Geometry: final body of the model. Coordinates: model frame, mm. A direction names the side the tool comes from. Give positions to 0.01 mm unless a question says otherwise; leave off trailing zeros. Write each loop counter-clockwise with the first axis right and the second up, starting at its lowest first coordinate (ties: lowest second). Pieces come first, ordered by that corner, then holes. Notation, with made-up numbers: M -38,11.25 L 13,11.25 A14 ccw 13,21.25 Z; hole C -8.75,55 d8. An arc over 180 degrees is marked long. Use a Markdown table: item, result. Add a question column.
1) Pin query (flat end, axial travel): pin 1 (1 mm diameter, centred on x = -36.5, z = 18.5, fed in from +Y); pin 2 (1.8 mm diameter, centred on x = 0.5, y = 0.5, fed in from +Z); pin 3 (1.6 mm diameter, centred on x = -37, y = -2, fed in from +Z). Return the tip coordinate at first contact, or that it passes through.
2) Section D-D on y = -12.5. Return the cut outline in (x, z), then the cut area to 3 significant figures.
3) Line query: line 1 (Y direction, x = -20, z = 24); line 2 (X direction, y = -23, z = 6); line 3 (Z direction, x = -0.5, y = 7). Output: solid intervals per line, ascending.
4) Set-up query: faces 1 (the flat face through (-1, 1, 0)), 2 (the flat face through (37.5, 1, 15)), 3 (the flat face through (-37, -20.029, 15)), 4 (the flat face through (0, 1, 2)), 5 (the flat face through (0, 0, 37)). Return all of +Z, -Z, +X, -X, +Y, -Y with unobstructed straight access to the full face (end or side cutting, diameter ignored); none if empty.
5) Draft query along X for faces 6 (the flat face through (-37.5, -0.6, 4.8)), 7 (the flat face through (-37, 12.126, 15)), 8 (the flat face through (35.5, 1, 15)). Return one class per face: +X half, -X half, draft (parallel to the pull), parting line (faces both ways), or undercut.
6) Section B-B on x = 0. Return the cut outline in (y, z).
7) Section C-C on y = 26. Return the cut outline in (x, z).
8) Section A-A on z = 3.5. Return the cut outline in (x, y), then the cut area to 3 significant figures.
Autodesk Inventor part; units mm, degrees
ref_plane "YZ Plane" through (0, 0, 0) normal (1, 0, 0) x (0, 1, 0)
ref_plane "XZ Plane" through (0, 0, 0) normal (0, 1, 0) x (-1, 0, 0)
ref_plane "XY Plane" through (0, 0, 0) normal (0, 0, 1) x (1, 0, 0)
sketch "Sketch1" plane through (0, 0, 0) normal (0, 0, 1) x (1, 0, 0)
  line L0 (-37.5, 45) -> (37.5, 45)
  line L1 (37.5, 45) -> (37.5, -45)
  line L2 (37.5, -45) -> (-37.5, -45)
  line L3 (-37.5, -45) -> (-37.5, 45)
  point P0 (0, 0)
  point P1 (0, -45)
  point P2 (0, 45)
  point P3 (-37.5, 0)
  dimension "d0" = 90
  dimension "d1" = 75
  dimension "d2" = 37.5
  dimension "d3" = 45
extrude "Extrusion1" add sketch "Sketch1" along normal blind 30
shell "Shell1" thickness 2 removed faces 0
sketch "Sketch2" plane through (-37.5, 45, 0) normal (0, 1, 0) x (1, 0, 0)
  circle A0 centre (42.5, -15) radius 2
  line L0 (75, 0) -> (0, 0)
  circle A1 centre (32.5, -15) radius 2
  line L1 (75, 0) -> (75, -30)
  point P0 (37.5, 0)
  point P1 (37.5, 0)
  dimension "d7" = 15
  dimension "d8" = 10
  dimension "d9" = 15
  dimension "d10" = 4
  dimension "d11" = 4
  dimension "d12" = 32.5
extrude "Extrusion2" add sketch "Sketch2" along normal blind 5
fillet "Fillet1" radius 2 1 edges at (3, 50, 15)
fillet "Fillet2" radius 2 1 edges at (-7, 50, 15)
chamfer "Chamfer1" distance 0.5 angle 45 1 edges at (3, 45, 15)
chamfer "Chamfer2" distance 0.5 angle 45 1 edges at (-7, 45, 15)
fillet "Fillet3" radius 0.5 1 edges at (3, 45.5, 15)
fillet "Fillet4" radius 0.5 1 edges at (-7, 45.5, 15)
sketch "Sketch3" plane through (0, 0, 30) normal (0, 0, 1) x (1, 0, 0)
  circle A0 centre (0, 0) radius 6
  dimension "d25" = 12
extrude "Extrusion3" add sketch "Sketch3" along normal blind 9
sketch "Sketch4" plane through (0, 0, 39) normal (0, 0, 1) x (1, 0, 0)
  circle A0 centre (0, 0) radius 1.75
  dimension "d28" = 3.5
extrude "Extrusion4" cut sketch "Sketch4" against normal blind 2
sketch "Sketch5" plane through (-37.5, 45, 0) normal (0, 1, 0) x (1, 0, 0)
  point P0 (37.5, 0)
sketch "Sketch6" plane through (-37.5, -45, 0) normal (-1, 0, 0) x (0, 0, 1)
  line L0 (25, 57.1263) -> (5, 57.1263)
  line L1 (5, 57.1263) -> (5, 24.9712)
  line L2 (5, 24.9712) -> (25, 24.9712)
  line L3 (25, 24.9712) -> (25, 57.1263)
  line L4 (30, 90) -> (30, 0)
  line L5 (0, 90) -> (0, 0)
  point P0 (0, 45)
  point P1 (25, 41.0487)
  dimension "d31" = 5
  dimension "d32" = 5
extrude "Extrusion5" cut sketch "Sketch6" against normal blind 2
sketch "Sketch7" plane through (-37.5, -45, 0) normal (-1, 0, 0) x (0, 0, 1)
  point P0 (0, 45)
equation "\"BendRadius\" = Thickness"
equation "\"BendReliefWidth\" = Thickness"
equation "\"BendReliefDepth\" = 0.5 * Thickness"
equation "\"CornerReliefSize\" = 4 * Thickness"
equation "\"MinimumRemnant\" = 2 * Thickness"
equation "\"TransitionRadius\" = BendRadius"
equation "\"JacobiRadiusSize\" = BendRadius"
equation "\"GapSize\" = Thickness"
properties part number "Utuh"
Found:
| question | item | result |
|---|---|---|
| 1 | pin 1 | y = 45 |
| 1 | pin 2 | z = 37 |
| 1 | pin 3 | z = 30 |
| 2 | outline | M -37.5,0 L 37.5,0 L 37.5,30 L -37.5,30 L -37.5,25 L -35.5,25 L -35.5,28 L 35.5,28 L 35.5,2 L -35.5,2 L -35.5,5 L -37.5,5 Z |
| 2 | area | 364 mm² |
| 3 | line 1 | -45 to -43, 43 to 45 |
| 3 | line 2 | -37.5 to -35.5, 35.5 to 37.5 |
| 3 | line 3 | 0 to 2, 28 to 30 |
| 4 | face 1 | -Z, +X, -X, +Y, -Y |
| 4 | face 2 | +Z, -Z, +X, +Y, -Y |
| 4 | face 3 | -X |
| 4 | face 4 | none |
| 4 | face 5 | +Z |
| 5 | face 6 | -X half |
| 5 | face 7 | draft |
| 5 | face 8 | undercut |
| 6 | outline | M -45,0 L 45,0 L 45,30 L 6,30 L 6,39 L 1.75,39 L 1.75,37 L -1.75,37 L -1.75,39 L -6,39 L -6,30 L -45,30 Z; hole M -43,2 L 43,2 L 43,28 L -43,28 Z |
| 7 | outline | M -37.5,0 L 37.5,0 L 37.5,30 L -37.5,30 Z; hole M -35.5,2 L 35.5,2 L 35.5,28 L -35.5,28 Z |
| 8 | outline | M -37.5,-45 L 37.5,-45 L 37.5,45 L -37.5,45 Z; hole M -35.5,-43 L 35.5,-43 L 35.5,43 L -35.5,43 Z |
| 8 | area | 644 mm² |
